from build123d import *

# Parameters (mm, degrees)
SKIZZE1_R                       = 45
AUFSATZ_LINEAR_AUSTRAGEN1_DEPTH = 50
SKIZZE2_R                       = 31.5
SKIZZE2_R_2                     = 15.75
SKIZZE2_R_3                     = 3
AUFSATZ_LINEAR_AUSTRAGEN2_DEPTH = 6.2
FASE1_SIZE                      = 1


with BuildPart() as part:
    # Skizze1 → Aufsatz-Linear austragen1 (new body)
    with BuildSketch(Plane(origin=(0, 0, 0), x_dir=(1, 0, 0), z_dir=(0, 1, 0))):
        with Locations(Location((0, 0, 0), (0, 0, 270))):
            Circle(SKIZZE1_R)
    extrude(amount=AUFSATZ_LINEAR_AUSTRAGEN1_DEPTH)

    # Skizze2 → Aufsatz-Linear austragen2 (add)
    with BuildSketch(Plane(origin=(0, 50, 0), x_dir=(1, 0, 0), z_dir=(0, 1, 0))):
        with Locations(Location((0, 0, 0), (0, 0, 90))):
            Circle(SKIZZE2_R)
        with Locations(Location((0, 0, 0), (0, 0, 90))):
            Circle(SKIZZE2_R_2, mode=Mode.SUBTRACT)
        with Locations(Location((17.67766953, 17.67766953, 0), (0, 0, 90))):
            Circle(SKIZZE2_R_3, mode=Mode.SUBTRACT)
        with Locations(Location((0, 25, 0), (0, 0, 90))):
            Circle(SKIZZE2_R_3, mode=Mode.SUBTRACT)
        with Locations(Location((17.67766953, -17.67766953, 0), (0, 0, 90))):
            Circle(SKIZZE2_R_3, mode=Mode.SUBTRACT)
        with Locations(Location((-17.67766953, -17.67766953, 0), (0, 0, 90))):
            Circle(SKIZZE2_R_3, mode=Mode.SUBTRACT)
        with Locations(Location((-17.67766953, 17.67766953, 0), (0, 0, 90))):
            Circle(SKIZZE2_R_3, mode=Mode.SUBTRACT)
    extrude(amount=AUFSATZ_LINEAR_AUSTRAGEN2_DEPTH)

    # Fase1
    fase1_edges = [part.edges().sort_by_distance(p)[0] for p in [
        (0, 56.2, 31.5),
        (0, 56.2, 15.75),
        (17.67766953, 56.2, -14.67766953),
        (0, 56.2, -22),
        (17.67766953, 56.2, 20.67766953),
        (-17.67766953, 56.2, 20.67766953),
        (-17.67766953, 56.2, -14.67766953),
        (0, 50, -45),
    ]]
    chamfer(fase1_edges, length=FASE1_SIZE)


solid = part.part
CAD build for the part. Positions are in the model's coordinates, mm. A direction names the side the tool comes from. Coordinates: 2 decimals unless noted, no trailing zeros. Loops run counter-clockwise (first coordinate to the right, second up) from the corner with the lowest first, then second, coordinate; pieces in that order, holes last. Notation, with made-up numbers: (38.5, 31.5) -> (52.5, 31.5) arc R15 cw to (52.5, 53.5) -> close; hole circle Ø5 at (38.5, -24). An arc over 180 degrees is marked (long way). One line per item, written item: value.
1. Drill centre lines: line 1 (Z direction, x = -18, y = 54); line 2 (Y direction, x = -32, z = 25); line 3 (Z direction, x = -28, y = 35.5). Where is each one in solid material? Low to high. Write a range as [from, to].
Answers:
line 1: z = [-25.85, -20.66], [-14.7, 14.7], [20.66, 25.85]
line 2: y = [0, 50]
line 3: z = [-35.23, 35.23]
2. Flat gauge pins, fed straight in: P1, Ø3, axis at x = -1.5, z = -1, coming from the +Y side; P2, Ø12, axis at x = -29, y = 38.5, coming from the -Z side; P3, Ø12, axis at x = 31.5, y = 33.5, coming from the +Z side. Where does each tip first touch, or does it go through?
Answers:
P1: stops at y = 50
P2: stops at z = -38.68
P3: stops at z = 37.08
3. Pull direction X, two halves, no side cores. Call faces 3 (the face through (-31.232, 52.564, 4.101)), 4 (the face through (13, 56.2, -13)), 5 (the face through (-18, 50, -18)): pulls with the +X half, pulls with the -X half, needs draft (parallel to the pull), parting line crosses it, or undercut.
Answers:
face 3: parting line crosses it
face 4: needs draft
face 5: undercut
4. Slice it at B-B on z = 0. Write the cut outline in (x, y), and give its area (3 significant figures).
Answers:
outline: (-45, 0) -> (45, 0) -> (45, 49) -> (44, 50) -> (31.5, 50) -> (31.5, 55.2) -> (30.5, 56.2) -> (16.75, 56.2) -> (15.75, 55.2) -> (15.75, 50) -> (-15.75, 50) -> (-15.75, 55.2) -> (-16.75, 56.2) -> (-30.5, 56.2) -> (-31.5, 55.2) -> (-31.5, 50) -> (-44, 50) -> (-45, 49) -> close
area: 4,690 mm^2
5. Slice it at C-C on y = 16.5. Write the cut outline in (x, z), and give its area (3 significant figures).
Answers:
outline: circle Ø90 at (0, 0)
area: 6,360 mm^2
6. Slice it at A-A on x = 0. Write the cut outline in (y, z).
Answers:
outline: (0, -45) -> (49, -45) -> (50, -44) -> (50, -31.5) -> (55.2, -31.5) -> (56.2, -30.5) -> (56.2, -29) -> (55.2, -28) -> (50, -28) -> (50, -22) -> (55.2, -22) -> (56.2, -21) -> (56.2, -16.75) -> (55.2, -15.75) -> (50, -15.75) -> (50, 15.75) -> (55.2, 15.75) -> (56.2, 16.75) -> (56.2, 30.5) -> (55.2, 31.5) -> (50, 31.5) -> (50, 44) -> (49, 45) -> (0, 45) -> close
7. Which spindle directions (+Z, -Z, +X, -X, +Y, -Y) get a long thin tool onto all of the face, cutting with end or side? Do faces 1 (the face through (-15.616, 52.564, 2.05)), 2 (the face through (-17.235, 24.157, 41.569)). Say none if no direction does.
Answers:
face 1: +Y
face 2: +Y, -Y
